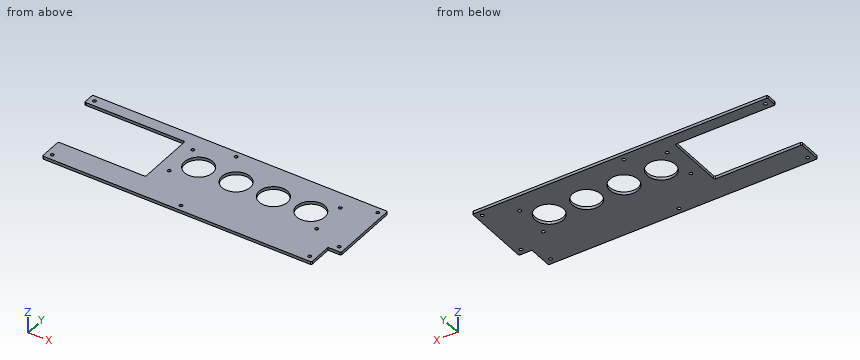
Autodesk Inventor part; units mm, degrees
ref_plane "YZ Plane" through (0, 0, 0) normal (1, 0, 0) x (0, 1, 0)
ref_plane "XZ Plane" through (0, 0, 0) normal (0, 1, 0) x (-1, 0, 0)
ref_plane "XY Plane" through (0, 0, 0) normal (0, 0, 1) x (1, 0, 0)
sketch "Sketch1" plane through (0, 0, 0) normal (0, 0, 1) x (1, 0, 0)
  line L0 (500, 160) -> (0, 160)
  line L1 (0, 160) -> (0, 140)
  line L2 (478, 0) -> (478, 42)
  line L3 (478, 42) -> (500, 42)
  line L4 (500, 42) -> (500, 160)
  line L5 (0, 0) -> (22, 0)
  line L6 (22, 0) -> (22, 40)
  line L7 (22, 0) -> (478, 0)
  line L8 (0, 42) -> (0, 0)
  line L9 (0, 140) -> (170, 140)
  line L10 (170, 140) -> (170, 40)
  line L11 (170, 40) -> (22, 40)
  line L12 (0, 56) -> (0, 42)
  dimension "d1" = 500
  dimension "d6" = 22
  dimension "d46" = 42
  dimension "d47" = 160
  dimension "d52" = 20
  dimension "d53" = 170
  dimension "d54" = 40
extrude "Extrusion1" add sketch "Sketch1" along normal blind 5
sketch "Sketch2" plane through (0, 0, 5) normal (0, 0, 1) x (1, 0, 0)
  circle A0 centre (32, 10) radius 2.75
  circle A1 centre (468, 10) radius 2.75
  circle A2 centre (10, 150) radius 2.75
  circle A3 centre (490, 150) radius 2.75
  circle A4 centre (490, 52) radius 2.75
  line L0 (500, 160) -> (0, 160)
  line L1 (500, 42) -> (500, 160)
  line L2 (478, 42) -> (500, 42)
  line L3 (478, 0) -> (478, 42)
  circle A5 centre (190, 130) radius 3.25
  circle A6 centre (440, 130) radius 3.25
  circle A7 centre (190, 70) radius 3.25
  circle A8 centre (440, 70) radius 3.25
  line L4 (0, 160) -> (0, 140)
  line L5 (22, 0) -> (478, 0)
  line L6 (22, 40) -> (22, 0)
  circle A9 centre (250, 150) radius 2.75
  circle A10 centre (250, 10) radius 2.75
  dimension "d9" = 5.5
  dimension "d10" = 10
  dimension "d12" = 10
  dimension "d13" = 10
  dimension "d14" = 10
  dimension "d15" = 10
  dimension "d16" = 10
  dimension "d20" = 5.5
  dimension "d21" = 5.5
  dimension "d22" = 5.5
  dimension "d23" = 5.5
  dimension "d34" = 60
  dimension "d35" = 60
  dimension "d38" = 30
  dimension "d39" = 6.5
  dimension "d40" = 6.5
  dimension "d41" = 6.5
  dimension "d42" = 6.5
  dimension "d43" = 30
  dimension "d55" = 70
  dimension "d56" = 190
  dimension "d57" = 190
  dimension "d58" = 10
  dimension "d59" = 10
  dimension "d60" = 10
  dimension "d61" = 10
  dimension "d62" = 70
  dimension "d63" = 10
  dimension "d64" = 10
  dimension "d65" = 5.5
  dimension "d66" = 5.5
  dimension "d67" = 250
  dimension "d68" = 250
fillet "Fillet1" radius 2 9 edges at (500, 160, 2.5) (500, 42, 2.5) (0, 160, 2.5) (478, 0, 2.5) (22, 0, 2.5) (22, 40, 2.5) (0, 140, 2.5) (170, 140, 2.5) (170, 40, 2.5)
hole "Hole6" at (10, 150, 5) at (250, 150, 5) at (490, 150, 5) at (490, 52, 5) at (468, 10, 5) at (250, 10, 5) at (32, 10, 5) at (190, 130, 5) at (190, 70, 5) at (440, 130, 5) at (440, 70, 5) direction (0, 0, -1) diameter 5.5 end through all
sketch "Sketch4" plane through (0, 0, 5) normal (0, 0, 1) x (1, 0, 0)
  circle A0 centre (220, 100) radius 24
  circle A1 centre (283.3333, 100) radius 24
  circle A2 centre (346.6667, 100) radius 24
  circle A3 centre (410, 100) radius 24
  circle A4 centre (190, 130) radius 2.75
  line L0 (207.2246, 100) -> (486.1087, 100) construction
  point P0 (0, 0)
  dimension "d115" = 30
  dimension "d116" = 30
  dimension "d117" = 63.3333
  dimension "d118" = 63.3333
  dimension "d119" = 63.3333
  dimension "d120" = 48
  dimension "d121" = 48
  dimension "d122" = 48
  dimension "d123" = 48
extrude "Extrusion2" cut sketch "Sketch4" against normal blind 10 contours A0 | A1 | A2 | A3
equation "\"d12\" = d10"
equation "\"d13\" = d10"
equation "\"d14\" = d10"
equation "\"d15\" = d10"
equation "\"d16\" = d10"
equation "\"d20\" = d9"
equation "\"d21\" = d9"
equation "\"d22\" = d9"
equation "\"d23\" = d9"
equation "\"d35\" = d34"
equation "\"d40\" = d39"
equation "\"d41\" = d39"
equation "\"d42\" = d39"
equation "\"d43\" = d38"
equation "\"d57\" = d56"
equation "\"d58\" = d10"
equation "\"d59\" = d10"
equation "\"d60\" = d10"
equation "\"d61\" = d10"
equation "\"d62\" = d55"
equation "\"d63\" = d10"
equation "\"d64\" = d10"
equation "\"d65\" = d9"
equation "\"d66\" = d9"
equation "\"d68\" = d67"
equation "\"d97\" = d9"
equation "\"d118\" = d117"
equation "\"d119\" = d117"
equation "\"d121\" = d120"
equation "\"d122\" = d120"
equation "\"d123\" = d120"
properties part number "BasePlate"
The model under review builds one solid part; all positions refer to its coordinate system, in mm. Give positions to 0.01 mm unless a question says otherwise; leave off trailing zeros. Write each loop counter-clockwise with the first axis right and the second up, starting at its lowest first coordinate (ties: lowest second). Pieces come first, ordered by that corner, then holes.
(1) Consider section A-A, the plane x = 410. Give the boundary of the cut face in (y, z).
(2) Consider section D-D, the plane x = 121.5. Give the boundary of the cut face in (y, z), and give its area (3 significant figures).
(3) Consider section C-C, the plane y = 107.5. Give the boundary of the cut face in (x, z).
(4) To check wall thickness, follow L1, parallel to Y at x = 250, z = 3.7; L2, parallel to Y at x = 117, z = 1.7; L3, parallel to Y at x = 468, z = 3.55. State the ranges of each line that lie inside material, in increasing order.
(5) Consider section B-B, the plane z = 1.35. Give the number of separate pieces and of enclosed holes in the cut face, and give its area (3 significant figures).
(6) For P1, Ø4, axis at x = 317.5, y = 39, coming from the -Z side; P2, Ø1.5, axis at x = 484, z = 3.5, coming from the -Y side; P3, Ø5, axis at x = 250, y = 150, coming from the -Z side (1 decimal); P4, Ø2.5, axis at y = 88.5, z = 2.5, coming from the -X side, all flat-tipped, find the tip position at first contact; note any pin that passes through.
Returned:
1. outline: (0, 0) - (76, 0) - (76, 5) - (0, 5) - close; (124, 0) - (160, 0) - (160, 5) - (124, 5) - close
2. outline: (0, 0) - (40, 0) - (40, 5) - (0, 5) - close; (140, 0) - (160, 0) - (160, 5) - (140, 5) - close
2. area: 300 mm2
3. outline: (170, 0) - (197.2, 0) - (197.2, 5) - (170, 5) - close; (242.8, 0) - (260.54, 0) - (260.54, 5) - (242.8, 5) - close; (306.13, 0) - (323.87, 0) - (323.87, 5) - (306.13, 5) - close; (369.46, 0) - (387.2, 0) - (387.2, 5) - (369.46, 5) - close; (432.8, 0) - (500, 0) - (500, 5) - (432.8, 5) - close
4. L1: y = 0 to 7.25, 12.75 to 147.25, 152.75 to 160
4. L2: y = 0 to 40, 140 to 160
4. L3: y = 0 to 7.25, 12.75 to 160
5. separate pieces: 1
5. enclosed holes: 15
5. area: 53,700 mm2
6. P1: stops at z = 0
6. P2: stops at y = 42
6. P3: passes through
6. P4: stops at x = 170
